The drawing under review shows one solid part. Ordinate dimensions are in mm from its lowest x, y, z. Give positions to 0.01 mm unless a question says otherwise; leave off trailing zeros. Loops run counter-clockwise (first coordinate to the right, second up) from the corner with the lowest first, then second, coordinate; pieces in that order, holes last.
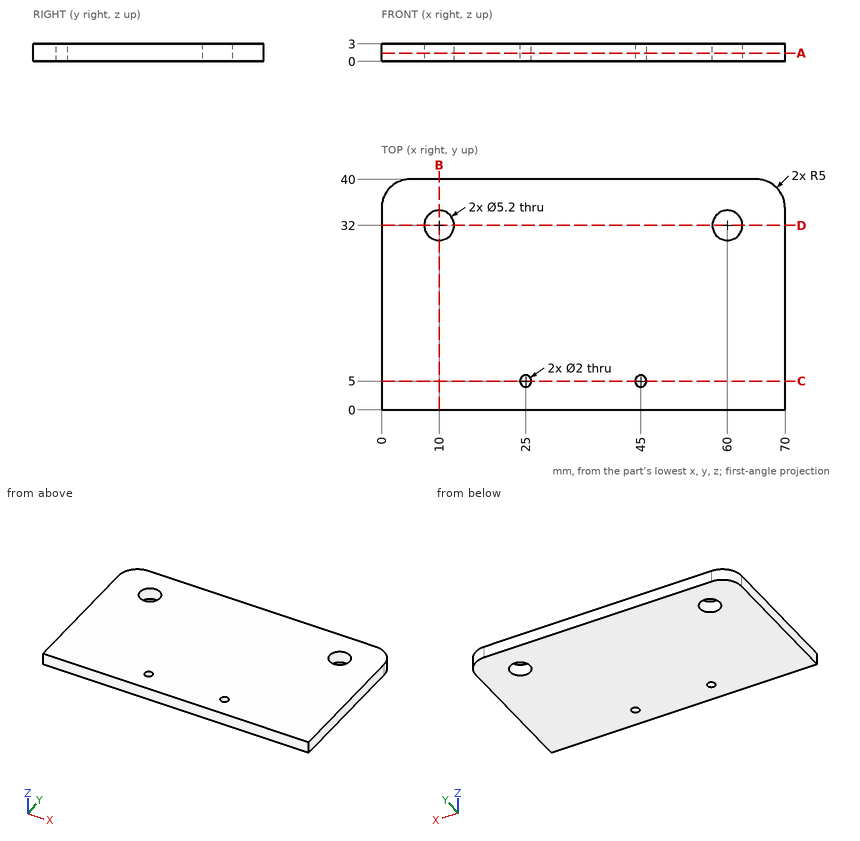
Item 1: Take a section at D-D on y = 32. Give the boundary of the cut face in (x, z).
Answer:
outline: (0, 0) - (7.4, 0) - (7.4, 3) - (0, 3) - close; (12.6, 0) - (57.4, 0) - (57.4, 3) - (12.6, 3) - close; (62.6, 0) - (70, 0) - (70, 3) - (62.6, 3) - close
Item 2: Take a section at A-A on z = 1.4. Give the boundary of the cut face in (x, y), and give its area (3 significant figures).
Answer:
outline: (0, 0) - (70, 0) - (70, 35) arc R5 ccw to (65, 40) - (5, 40) arc R5 ccw to (0, 35) - close; hole circle Ø5.2 at (10, 32); hole circle Ø2 at (25, 5); hole circle Ø2 at (45, 5); hole circle Ø5.2 at (60, 32)
area: 2,740 mm2
Item 3: Take a section at C-C on y = 5. Give the boundary of the cut face in (x, z).
Answer:
outline: (0, 0) - (24, 0) - (24, 3) - (0, 3) - close; (26, 0) - (44, 0) - (44, 3) - (26, 3) - close; (46, 0) - (70, 0) - (70, 3) - (46, 3) - close
Item 4: For L1, parallel to X at y = 5, z = 1.05; L2, parallel to Y at x = 45, z = 0.75; L3, parallel to Y at x = 60, z = 1.8, list the stretches that pass through material, from the lowest coordinate up.
Answer:
L1: x = 0 to 24, 26 to 44, 46 to 70
L2: y = 0 to 4, 6 to 40
L3: y = 0 to 29.4, 34.6 to 40
Item 5: Take a section at B-B on x = 10. Give the boundary of the cut face in (y, z).
Answer:
outline: (0, 0) - (29.4, 0) - (29.4, 3) - (0, 3) - close; (34.6, 0) - (40, 0) - (40, 3) - (34.6, 3) - close
